Read the model definition and answer for the solid it produces. Units are mm, in the model's axes. Face numbers are marked on the shaded views. A direction names the side the tool comes from. Coordinates: 2 decimals unless noted, no trailing zeros. Order: outer loops, then holes, each group sorted by start corner. A loop starts at its lowest first (then second) coordinate and runs counter-clockwise, first axis right, second up. Notation, with made-up numbers: (14, 11.5) - (50, 11.5) arc R20 ccw to (50, 25.5) - close; hole circle Ø1 at (78.5, -18.75). An arc over 180 degrees is marked (long way). Write item = value, one per line.
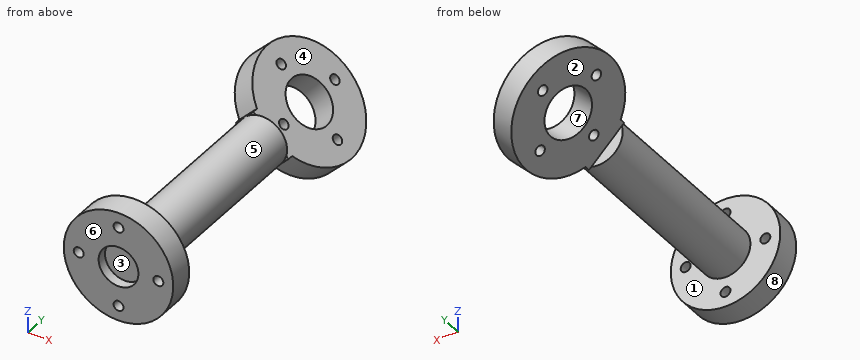
Autodesk Inventor part; units mm, degrees
ref_plane "YZ Plane" through (0, 0, 0) normal (1, 0, 0) x (0, 1, 0)
ref_plane "XZ Plane" through (0, 0, 0) normal (0, 1, 0) x (-1, 0, 0)
sketch "Esquisse1" plane through (0, 0, 0) normal (0, 1, 0) x (-1, 0, 0)
  circle A0 centre (0, 0) radius 11
  line L0 (0, 0) -> (-8, 0) construction
  circle A1 centre (-8, 0) radius 1
  circle A2 centre (0, -8) radius 1
  circle A3 centre (8, 0) radius 1
  circle A4 centre (0, 8) radius 1
  circle A5 centre (0, 0) radius 4
  dimension "d0" = 22
  dimension "d1" = 8
  dimension "d2" = 2
  dimension "d5" = 360
  dimension "d7" = 8
extrude "Extrusion1" add sketch "Esquisse1" along normal blind 5
sketch "Esquisse2" plane through (0, 5, 0) normal (0, 1, 0) x (1, 0, 0)
  circle A0 centre (0, 0) radius 4
extrude "Extrusion2" add sketch "Esquisse2" against normal blind 3
sketch "Esquisse3" plane through (0, 5, 0) normal (0, 1, 0) x (1, 0, 0)
  circle A0 centre (0, 0) radius 11
  circle A1 centre (0, 0) radius 5
  dimension "d12" = 10
extrude "Extrusion3" add sketch "Esquisse3" along normal blind 40 contours A1
ref_plane "Plan de construction1" through (0, 0, 0) normal (0.7071, 0, 0.7071) x (0, 1, 0)
sketch "Esquisse4" plane through (0, 0, 0) normal (0.7071, 0, 0.7071) x (0, 1, 0)
  line L0 (0, 0) -> (5, 0) construction
  line L1 (5, 0) -> (5, -5) construction
  line L2 (5, 0) -> (5, 5)
  line L3 (5, 0) -> (5, -5)
  line L4 (0, 0) -> (45, 0) construction
  line L5 (45, 0) -> (57, 0) construction
  circle A0 centre (57, 0) radius 12
  circle A1 centre (57, 0) radius 8 construction
  line L6 (0, 0) -> (45, 0) construction
  line L7 (45, 0) -> (57, 0) construction
  circle A2 centre (65, 0) radius 1
  circle A3 centre (57, 8) radius 1
  circle A4 centre (49, 0) radius 1
  circle A5 centre (57, -8) radius 1
  circle A6 centre (57, 0) radius 5
  line L8 (46.0913, 5) -> (45, 5)
  line L9 (45, 5) -> (45, 0)
  line L10 (45, -5) -> (46.0913, -5)
  line L11 (45, 0) -> (45, -5)
  dimension "d53" = 16
  dimension "d36" = 45
  dimension "d52" = 12
  dimension "d54" = 2
  dimension "d57" = 360
  dimension "d59" = 10
extrude "Extrusion6" add sketch "Esquisse4" along normal mid plane 5
properties part number "neck_v2"
1) The part is cut by section C-C (y = 36). Determine the outline of the cut face in (x, z), and give its area (3 significant figures).
Returned:
outline = circle Ø10 at (0, 0)
area = 78.5 mm^2
2) The part is cut by section A-A (z = 0). Count the separate pieces of the cut face and the enclosed holes in it, and give its area (3 significant figures).
Returned:
separate_pieces = 4
enclosed_holes = 2
area = 567 mm^2
3) Flat-ended cylindrical pins translate along their axes: pin 1 Ø8 at (y, z) = (60, -2) entering from -X; pin 2 Ø4 at (y, z) = (31.5, -4.5) entering from -X; pin 3 Ø2.5 at (x, z) = (-8, 0) entering from +Y; pin 4 Ø1.8 at (x, z) = (8, 0) entering from -Y. Find the tip coordinate at first contact, or state that the pin passes through.
Returned:
pin_1 = -5.54
pin_2 = -4.33
pin_3 = 5
pin_4 = through
4) Determine the mould class of the marked faces 5, 6, 7 and 8 for opening direction Y: pulls with the +Y half, pulls with the -Y half, needs draft (parallel to the pull), parting line crosses it, or undercut.
Returned:
face_5 = undercut
face_6 = pulls with the -Y half
face_7 = undercut
face_8 = needs draft
5) Straight lines are drawn through the part: line 1 along Z through (x, y) = (0, 1.45); line 2 along Z through (x, y) = (0, 2.45); line 3 along Y through (x, z) = (1.5, -5). For each, find the intervals that lie inside material, in ascending order. Write a range as from..to.
Returned:
line_1 = -11..-9, -7..-4, 4..7, 9..11
line_2 = -11..-9, -7..7, 9..11
line_3 = 0..5, 45..55.03, 58.97..68.08
6) For the marked faces 1, 2, 3 and 4, determine the directions among +Z, -Z, +X, -X, +Y, -Y from which every point of the face is accessible in a straight line to the end or side of a thin tool.
Returned:
face_1 = none
face_2 = -Z, -X, +Y
face_3 = -Y
face_4 = +Z, +X, +Y
